Build history of the part. All positions in model axes, mm. Face numbers are marked on the shaded views. Round coordinates to 2 decimals unless told otherwise and drop trailing zeros. Write each loop counter-clockwise with the first axis right and the second up, starting at its lowest first coordinate (ties: lowest second). Pieces come first, ordered by that corner, then holes. Notation, with made-up numbers: M 82.25,-35.75 L 101.25,-35.75 A29 cw 101.25,-7.75 Z; hole C 17,-38.75 d11. An arc over 180 degrees is marked long. Use a Markdown table: item, result.
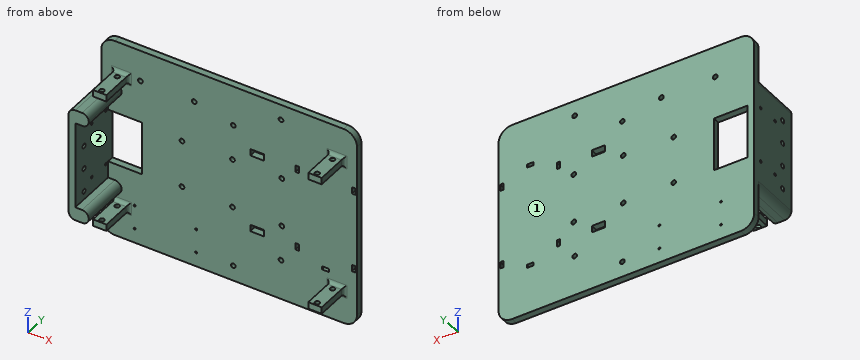
from build123d import *

# Parameters (mm, degrees)
BOSS_EXTRUDE1_DEPTH = 5
SKETCH2_R           = 1.75
SKETCH2_R_2         = 0.75
SKETCH2_W           = 10
SKETCH2_H           = 5
SKETCH2_W_2         = 2.5
SKETCH2_W_3         = 25
SKETCH2_H_2         = 40
SKETCH2_W_4         = 5
SKETCH2_H_3         = 2.5
CUT_EXTRUDE1_DEPTH  = 122.140414396
SKETCH6_W           = 10
SKETCH6_H           = 5
BOSS_EXTRUDE3_DEPTH = 25
SKETCH7_R           = 1.75
CUT_EXTRUDE3_DEPTH  = 158.023087474
FILLET1_R           = 2.5
MIRROR2_START       = -55
MIRROR2_OUTLINE_R   = 1.75
MIRROR2_DEPTH       = 10
MIRROR2_START_2     = 45
MIRROR2_2_OUTLINE_R = 1.75
MIRROR2_2_DEPTH     = 10
MIRROR2_START_3     = -87.5
MIRROR2_3_DEPTH     = 175.5
SKETCH8_W           = 10
SKETCH8_H           = 10
BOSS_EXTRUDE4_DEPTH = 37.5
SKETCH9_W           = 85
SKETCH9_H           = 37.5
BOSS_EXTRUDE8_DEPTH = 5
SKETCH10_R          = 1.75
SKETCH10_R_2        = 1
CUT_EXTRUDE4_DEPTH  = 204.116345969
FILLET2_R           = 5


with BuildPart() as part:
    # Sketch1 → Boss-Extrude1 (new body)
    with BuildSketch(Plane(origin=(0, 0, 0), x_dir=(1, 0, 0), z_dir=(0, 1, 0))):
        with BuildLine():
            Line((-85, -75), (85, -75))
            ThreePointArc((85, -75), (92.071067812, -72.071067812), (95, -65))
            Line((95, -65), (95, 65))
            ThreePointArc((95, 65), (92.071067812, 72.071067812), (85, 75))
            Line((85, 75), (-85, 75))
            ThreePointArc((-85, 75), (-92.071067812, 72.071067812), (-95, 65))
            Line((-95, 65), (-95, -65))
            ThreePointArc((-95, -65), (-92.071067812, -72.071067812), (-85, -75))
        make_face()
    extrude(amount=BOSS_EXTRUDE1_DEPTH)

    # Sketch2 → Cut-Extrude1 (cut, through all)
    with BuildSketch(Plane(origin=(0, 5, 0), x_dir=(1, 0, 0), z_dir=(0, 1, 0))):
        with Locations(Location((-66, -51.75, 0), (0, 0, 270))):
            Circle(SKETCH2_R)
        with Locations(Location((-26, -51.75, 0), (0, 0, 270))):
            Circle(SKETCH2_R)
        with Locations(Location((-35.1, 17.6, 0), (0, 0, 270))):
            Circle(SKETCH2_R)
        with Locations(Location((-35.1, -17.6, 0), (0, 0, 270))):
            Circle(SKETCH2_R)
        with Locations(Location((2.400579028, 18.349420972, 0), (0, 0, 270))):
            Circle(SKETCH2_R)
        with Locations(Location((39.099420972, 18.349420972, 0), (0, 0, 270))):
            Circle(SKETCH2_R)
        with Locations(Location((39.099420972, -18.349420972, 0), (0, 0, 270))):
            Circle(SKETCH2_R)
        with Locations(Location((2.400579028, -18.349420972, 0), (0, 0, 270))):
            Circle(SKETCH2_R)
        with Locations(Location((3.011718317, -45.011311623, 0), (0, 0, 270))):
            Circle(SKETCH2_R)
        with Locations(Location((38.488281683, -63.488688377, 0), (0, 0, 270))):
            Circle(SKETCH2_R)
        with Locations(Location((38.488281683, 45.011311623, 0), (0, 0, 270))):
            Circle(SKETCH2_R)
        with Locations(Location((3.011718317, 63.488688377, 0), (0, 0, 270))):
            Circle(SKETCH2_R)
        with Locations(Location((-70.26, 64.19, 0), (0, 0, 270))):
            Circle(SKETCH2_R_2)
        with Locations(Location((-70.26, 46.41, 0), (0, 0, 270))):
            Circle(SKETCH2_R_2)
        with Locations(Location((-24.54, 64.19, 0), (0, 0, 270))):
            Circle(SKETCH2_R_2)
        with Locations(Location((-24.54, 46.41, 0), (0, 0, 270))):
            Circle(SKETCH2_R_2)
        with Locations((20.75, -29.25)):
            Rectangle(SKETCH2_W, SKETCH2_H)
        with Locations((50.5, 30)):
            Rectangle(SKETCH2_W_2, SKETCH2_H)
        with Locations((50.5, -30)):
            Rectangle(SKETCH2_W_2, SKETCH2_H)
        with Locations((92.5, -30)):
            Rectangle(SKETCH2_W_2, SKETCH2_H)
        with Locations((92.5, 30)):
            Rectangle(SKETCH2_W_2, SKETCH2_H)
        with Locations((-77.5, 0)):
            Rectangle(SKETCH2_W_3, SKETCH2_H_2)
        with Locations((20.75, 29.25)):
            Rectangle(SKETCH2_W, SKETCH2_H)
        with Locations((71.5, -38.75)):
            Rectangle(SKETCH2_W_4, SKETCH2_H_3)
        with Locations((71.5, 38.75)):
            Rectangle(SKETCH2_W_4, SKETCH2_H_3)
    extrude(amount=-CUT_EXTRUDE1_DEPTH, mode=Mode.SUBTRACT)

    # Sketch6 → Boss-Extrude3 (add)
    with BuildSketch(Plane.XZ):
        with Locations((-80, 50)):
            Rectangle(SKETCH6_W, SKETCH6_H)
    extrude(amount=BOSS_EXTRUDE3_DEPTH)

    # Sketch7 → Cut-Extrude3 (cut, through all)
    with BuildSketch(Plane(origin=(0, 0, 47.5), x_dir=(-1, 0, 0), z_dir=(0, 0, -1))):
        with Locations((80, -22.5)):
            Circle(SKETCH7_R)
        with Locations((80, -5)):
            Circle(SKETCH7_R)
    extrude(amount=-CUT_EXTRUDE3_DEPTH, mode=Mode.SUBTRACT)

    # Fillet1
    fillet1_edges = [part.edges().sort_by_distance(p)[0] for p in [
        (-75, 0, 50),
        (-80, 0, 52.5),
        (-85, 0, 50),
        (-80, 0, 47.5),
    ]]
    fillet(fillet1_edges, radius=FILLET1_R)

    # Mirror2: read off the stored shape, not the designer's step
    # Mirror2 outline → Mirror2 (add)
    # profile 1 of 2: a face of its own
    with BuildSketch(Plane.XY.offset(MIRROR2_START)):
        with BuildLine():
            Line((87.5, 0), (72.5, 0))
            ThreePointArc((72.5, 0), (74.267766953, -0.732233047), (75, -2.5))
            Line((75, -2.5), (75, -25))
            Line((75, -25), (85, -25))
            Line((85, -25), (85, -2.5))
            ThreePointArc((85, -2.5), (85.732233047, -0.732233047), (87.5, 0))
        make_face()
        with Locations((80, -22.5)):
            Circle(MIRROR2_OUTLINE_R, mode=Mode.SUBTRACT)
        with Locations((80, -5)):
            Circle(MIRROR2_OUTLINE_R, mode=Mode.SUBTRACT)
    # profile 2 of 2: a face of its own
    with BuildSketch(Plane.XY.offset(MIRROR2_START)):
        with BuildLine():
            Line((-75, -25), (-75, -2.5))
            ThreePointArc((-75, -2.5), (-74.267766953, -0.732233047), (-72.5, 0))
            Line((-72.5, 0), (-87.5, 0))
            ThreePointArc((-87.5, 0), (-85.732233047, -0.732233047), (-85, -2.5))
            Line((-85, -2.5), (-85, -25))
            Line((-85, -25), (-75, -25))
        make_face()
        with Locations((-80, -22.5)):
            Circle(MIRROR2_OUTLINE_R, mode=Mode.SUBTRACT)
        with Locations((-80, -5)):
            Circle(MIRROR2_OUTLINE_R, mode=Mode.SUBTRACT)
    extrude(amount=MIRROR2_DEPTH)

    # Mirror2 2 outline → Mirror2 2 (add)
    with BuildSketch(Plane.XY.offset(MIRROR2_START_2)):
        with BuildLine():
            Line((87.5, 0), (72.5, 0))
            ThreePointArc((72.5, 0), (74.267766953, -0.732233047), (75, -2.5))
            Line((75, -2.5), (75, -25))
            Line((75, -25), (85, -25))
            Line((85, -25), (85, -2.5))
            ThreePointArc((85, -2.5), (85.732233047, -0.732233047), (87.5, 0))
        make_face()
        with Locations((80, -22.5)):
            Circle(MIRROR2_2_OUTLINE_R, mode=Mode.SUBTRACT)
        with Locations((80, -5)):
            Circle(MIRROR2_2_OUTLINE_R, mode=Mode.SUBTRACT)
    extrude(amount=MIRROR2_2_DEPTH)

    # Mirror2 3 outline → Mirror2 3 (cut)
    with BuildSketch(Plane.YZ.offset(MIRROR2_START_3)):
        with BuildLine():
            Line((-25, 55), (-25, 52.5))
            Line((-25, 52.5), (-2.5, 52.5))
            ThreePointArc((-2.5, 52.5), (-0.732233047, 53.232233047), (0, 55))
            Line((0, 55), (-25, 55))
        make_face()
        with BuildLine():
            Line((-2.5, 47.5), (-25, 47.5))
            Line((-25, 47.5), (-25, 45))
            Line((-25, 45), (0, 45))
            ThreePointArc((0, 45), (-0.732233047, 46.767766953), (-2.5, 47.5))
        make_face()
        with BuildLine():
            Line((-25, -47.5), (-2.5, -47.5))
            ThreePointArc((-2.5, -47.5), (-0.732233047, -46.767766953), (0, -45))
            Line((0, -45), (-25, -45))
            Line((-25, -45), (-25, -47.5))
        make_face()
        with BuildLine():
            Line((-2.5, -52.5), (-25, -52.5))
            Line((-25, -52.5), (-25, -55))
            Line((-25, -55), (0, -55))
            ThreePointArc((0, -55), (-0.732233047, -53.232233047), (-2.5, -52.5))
        make_face()
    extrude(amount=MIRROR2_3_DEPTH, mode=Mode.SUBTRACT)

    # Sketch8 → Boss-Extrude4 (add)
    with BuildSketch(Plane.XZ):
        with Locations((-85, 37.5)):
            Rectangle(SKETCH8_W, SKETCH8_H)
        with Locations((-85, -37.5)):
            Rectangle(SKETCH8_W, SKETCH8_H)
    extrude(amount=BOSS_EXTRUDE4_DEPTH)

    # Sketch9 → Boss-Extrude8 (add)
    with BuildSketch(Plane.ZY.offset(90)):
        with Locations((0, -18.75)):
            Rectangle(SKETCH9_W, SKETCH9_H)
    extrude(amount=BOSS_EXTRUDE8_DEPTH)

    # Sketch10 → Cut-Extrude4 (cut, through all)
    with BuildSketch(Plane(origin=(-90, 0, 0), x_dir=(0, 0, -1), z_dir=(1, 0, 0))):
        with Locations((-26.25, -27.5)):
            Circle(SKETCH10_R)
        with Locations((-8.75, -27.5)):
            Circle(SKETCH10_R)
        with Locations((8.75, -27.5)):
            Circle(SKETCH10_R)
        with Locations((26.25, -27.5)):
            Circle(SKETCH10_R)
        with Locations((-20.65, -2.5)):
            Circle(SKETCH10_R_2)
        with Locations((-20.65, -18.8)):
            Circle(SKETCH10_R_2)
        with Locations((20.65, -2.5)):
            Circle(SKETCH10_R_2)
        with Locations((20.65, -18.8)):
            Circle(SKETCH10_R_2)
    extrude(amount=-CUT_EXTRUDE4_DEPTH, mode=Mode.SUBTRACT)

    # Fillet2
    fillet2_edges = [part.edges().sort_by_distance(p)[0] for p in [
        (-80, -18.75, -42.5),
        (-80, -18.75, -32.5),
        (-95, -18.75, -42.5),
        (-95, -18.75, 42.5),
        (-80, -18.75, 42.5),
        (-80, -18.75, 32.5),
    ]]
    fillet(fillet2_edges, radius=FILLET2_R - 0.0001)  # a hair under: the kernel refuses the full size


solid = part.part
Q1. Two-plate mould, pull along Z, no slides. Class the marked faces 1 and 2: +Z half, -Z half, draft (parallel to the pull), parting line (faces both ways), or undercut.
Response values:
| item | result |
|---|---|
| face 1 | draft |
| face 2 | undercut |
Q2. Drop flat-ended pins along their axis: P1, Ø1, axis at y = -25, z = 25, coming from the +X side; P2, Ø6, axis at x = 0, z = -20.5, coming from the -Y side; P3, Ø4, axis at x = -88.5, y = -11.5, coming from the +Z side; P4, Ø2, axis at x = -35.1, z = 17.6, coming from the -Y side. Give the stop position or say it passes through.
Response values:
| item | result |
|---|---|
| P1 | stops at x = -90 |
| P2 | stops at y = 0 |
| P3 | stops at z = 42.5 |
| P4 | passes through |
Q3. Drill centre lines: L1, parallel to X at y = 3.25, z = 51.75; L2, parallel to X at y = 2, z = 51; L3, parallel to Y at x = 53, z = -27. Where is each one in solid material? Low to high.
Response values:
| item | result |
|---|---|
| L1 | x = -95 to -67.75, -64.25 to -27.75, -24.25 to 95 |
| L2 | x = -95 to -67.58, -64.42 to -27.58, -24.42 to 95 |
| L3 | y = 0 to 5 |
Q4. Cut at B-B on x = -42. Give the cut face in (y, z), and give its area (3 significant figures).
Response values:
| item | result |
|---|---|
| outline | M 0,-75 L 5,-75 L 5,75 L 0,75 Z |
| area | 750 mm2 |
